Design review of the part built by this model. Coordinates are the model's own, in mm. Face numbers are marked on the shaded views. A direction names the side the tool comes from. Coordinates: 2 decimals unless noted, no trailing zeros. Loops run counter-clockwise (first coordinate to the right, second up) from the corner with the lowest first, then second, coordinate; pieces in that order, holes last. Notation, with made-up numbers: (-9, -3) -> (23, -3) arc R15 ccw to (23, 8) -> close; hole circle Ø11 at (82, 87.5). An arc over 180 degrees is marked (long way). Use CSV: the item, a comma, the result in double quotes.
```python
from build123d import *

# Parameters (mm, degrees)
ESQUISSE1_R             = 2
BOSS_EXTRU_1_DEPTH      = 8
ESQUISSE2_R             = 2
ENL_V_MAT_EXTRU_1_DEPTH = 20
CONG_1_R                = 4


with BuildPart() as part:
    # Esquisse1 → Boss.-Extru.1 (new body)
    with BuildSketch(Plane.XY):
        with BuildLine():
            Line((14.823672032, -22.72937471), (6.823672032, -22.72937471))
            Line((6.823672032, -22.72937471), (6.823672032, -5.72937471))
            ThreePointArc((6.823672032, -5.72937471), (3.664545235, -5.455042233), (0.599995261, -4.640257669))
            ThreePointArc((0.599995261, -4.640257669), (-0.7167539, -6.768921529), (-1.176327968, -9.22937471))
            ThreePointArc((-1.176327968, -9.22937471), (-5.176327968, -13.22937471), (-9.176327968, -9.22937471))
            ThreePointArc((-9.176327968, -9.22937471), (-8.40967046, -4.525117147), (-6.189038967, -0.307701027))
            ThreePointArc((-6.189038967, -0.307701027), (-7.431435725, 1.079388257), (-8.526663538, 2.58539039))
            ThreePointArc((-8.526663538, 2.58539039), (-7.361562867, 8.12096086), (-1.825992398, 6.955860189))
            ThreePointArc((-1.825992398, 6.955860189), (1.905132594, 3.517167866), (6.823672032, 2.27062529))
            Line((6.823672032, 2.27062529), (14.823672032, 2.27062529))
            Line((14.823672032, 2.27062529), (14.823672032, -22.72937471))
        make_face()
        with Locations((-5.176327968, 4.77062529)):
            Circle(ESQUISSE1_R, mode=Mode.SUBTRACT)
        with Locations((6.823672032, -1.72937471)):
            Circle(ESQUISSE1_R, mode=Mode.SUBTRACT)
        with Locations((-5.176327968, -9.22937471)):
            Circle(ESQUISSE1_R, mode=Mode.SUBTRACT)
    extrude(amount=BOSS_EXTRU_1_DEPTH)

    # Esquisse2 → Enlèv. mat.-Extru.1 (cut)
    with BuildSketch(Plane.XZ.offset(22.72937471)):
        with Locations((10.823672032, 4)):
            Circle(ESQUISSE2_R)
    extrude(amount=-ENL_V_MAT_EXTRU_1_DEPTH, mode=Mode.SUBTRACT)

    # Congé1
    cong_1_edges = [part.edges().sort_by_distance(p)[0] for p in [
        (-6.189038967, -0.307701027, 4),
        (0.599995261, -4.640257669, 4),
        (6.823672032, -5.72937471, 4),
        (14.823672032, 2.27062529, 4),
    ]]
    fillet(cong_1_edges, radius=CONG_1_R)


solid = part.part
```
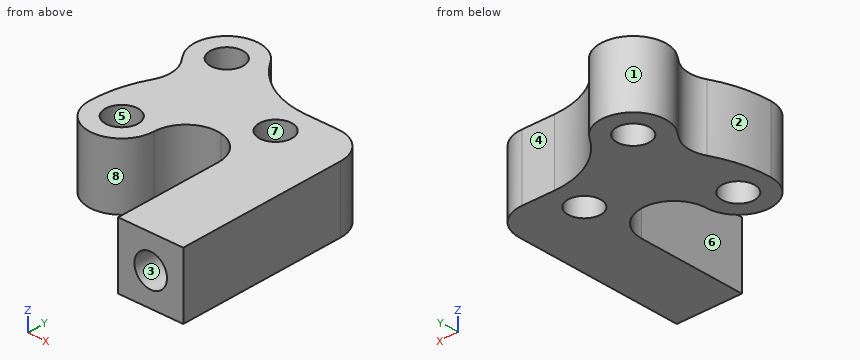
Item 1: Add section B-B (y = -18). Give the boundary of the cut face in (x, z), then the cut area to 3 significant figures.
Checked values:
outline,"(6.82, 0) -> (14.82, 0) -> (14.82, 8) -> (6.82, 8) -> close; hole circle Ø4 at (10.82, 4)"
area,"51.4 mm^2"
Item 2: Clearance check with flat-ended pins moving along their axes: pin 1 (1.2 mm diameter, centred on x = 11.5, z = 5, fed in from -Y); pin 2 (2 mm diameter, centred on x = 8.5, z = 4.5, fed in from +Y). State where each tip first meets the part, or that it passes through.
Checked values:
pin 1,"y = -2.73"
pin 2,"y = 2.27"
Item 3: Machinability: for the marked faces 1, 2, 3 and 4, which of the approach directions +Z, -Z, +X, -X, +Y, -Y give a long, thin tool a straight path to every point of the face, cutting with its end or side? Answer none if there is none.
Checked values:
face 1,"+Z, -Z"
face 2,"+Z, -Z, -X"
face 3,"-Y"
face 4,"+Z, -Z, +X, +Y"
Item 4: Add section A-A (x = 6). Give the boundary of the cut face in (y, z), then the cut area to 3 significant figures.
Checked values:
outline,"(-6.94, 0) -> (-3.55, 0) -> (-3.55, 8) -> (-6.94, 8) -> close; (0.09, 0) -> (2.3, 0) -> (2.3, 8) -> (0.09, 8) -> close"
area,"44.8 mm^2"
Item 5: Add section C-C (y = 6). Give the boundary of the cut face in (x, z), then the cut area to 3 significant figures.
Checked values:
outline,"(-8.98, 0) -> (-6.75, 0) -> (-6.75, 8) -> (-8.98, 8) -> close; (-3.6, 0) -> (-1.12, 0) -> (-1.12, 8) -> (-3.6, 8) -> close"
area,"37.7 mm^2"
Item 6: Add section D-D (z = 1.5). State how many separate pieces and enclosed holes the cut face has, then the cut area to 3 significant figures.
Checked values:
separate pieces,"1"
enclosed holes,"3"
area,"386 mm^2"
Item 7: To check wall thickness, follow line 1 along Y through (x, z) = (-6, 3.5); line 2 along Y through (x, z) = (-5.75, 1.75); line 3 along X through (y, z) = (-5, 3). State the ranges of each line that lie inside material, in increasing order.
Checked values:
line 1,"-13.14 to -11.05, -7.41 to 2.95, 6.59 to 8.68"
line 2,"-13.19 to -11.15, -7.31 to 2.85, 6.69 to 8.73"
line 3,"-8.56 to 9.09, 12.56 to 14.82"
Item 8: Draft analysis for pull direction Y (two halves, no side actions). For the marked faces 5, 6, 7 and 8, state which applies: pulls with the +Y half, pulls with the -Y half, needs draft (parallel to the pull), parting line crosses it, or undercut.
Checked values:
face 5,"undercut"
face 6,"needs draft"
face 7,"undercut"
face 8,"pulls with the -Y half"
